from build123d import *

# Parameters (mm, degrees)
SKETCH_W                     = 43.9
SKETCH_H                     = 43.9
SKETCH_W_2                   = 40.7
SKETCH_H_2                   = 40.7
PAD_DEPTH                    = 135
SKETCH001_W                  = 43.9
SKETCH001_H                  = 43.9
PAD001_DEPTH                 = 1.6
PAD002_DEPTH                 = 11.5
PAD002_POLARPATTERN_2_DEPTH  = 11.5
PAD002_POLARPATTERN_3_DEPTH  = 11.5
PAD002_POLARPATTERN_4_DEPTH  = 11.5
SKETCH003_W                  = 43.9
SKETCH003_H                  = 43.9
SKETCH003_W_2                = 35.9
SKETCH003_H_2                = 35.9
PAD003_DEPTH                 = 3.2
PAD004_DEPTH                 = 20
POCKET_DEPTH                 = 21.6
PAD004_LINEARPATTERN_2_DEPTH = 20
POCKET_LINEARPATTERN_2_DEPTH = 21.6


with BuildPart() as part:
    # Sketch → Pad (new body)
    with BuildSketch(Plane.XZ):
        Rectangle(SKETCH_W, SKETCH_H)
        Rectangle(SKETCH_W_2, SKETCH_H_2, mode=Mode.SUBTRACT)
    extrude(amount=PAD_DEPTH)

    # Sketch001 → Pad001 (join)
    with BuildSketch(Plane.XZ):
        Rectangle(SKETCH001_W, SKETCH001_H)
    extrude(amount=-PAD001_DEPTH)

    # Sketch002 → Pad002 (join)
    with BuildSketch(Plane.XZ.offset(135)):
        with BuildLine():
            ThreePointArc((-14.31, 21.95), (-12.21, 19.85), (-10.11, 21.95))
            Line((-14.31, 21.95), (-10.11, 21.95))
        make_face()
    pad002 = extrude(amount=-PAD002_DEPTH)

    # Sketch002 PolarPattern 2 → Pad002 PolarPattern 2 (add)
    with BuildSketch(Plane(origin=(0, -135, 0), x_dir=(0, 0, 1), z_dir=(0, -1, 0))):
        with BuildLine():
            ThreePointArc((-14.31, 21.95), (-12.21, 19.85), (-10.11, 21.95))
            Line((-14.31, 21.95), (-10.11, 21.95))
        make_face()
    pad002_polarpattern_2 = extrude(amount=-PAD002_POLARPATTERN_2_DEPTH)

    # Sketch002 PolarPattern 3 → Pad002 PolarPattern 3 (add)
    with BuildSketch(Plane(origin=(0, -135, 0), x_dir=(-1, 0, 0), z_dir=(0, -1, 0))):
        with BuildLine():
            ThreePointArc((-14.31, 21.95), (-12.21, 19.85), (-10.11, 21.95))
            Line((-14.31, 21.95), (-10.11, 21.95))
        make_face()
    pad002_polarpattern_3 = extrude(amount=-PAD002_POLARPATTERN_3_DEPTH)

    # Sketch002 PolarPattern 4 → Pad002 PolarPattern 4 (add)
    with BuildSketch(Plane(origin=(0, -135, 0), x_dir=(0, 0, -1), z_dir=(0, -1, 0))):
        with BuildLine():
            ThreePointArc((-14.31, 21.95), (-12.21, 19.85), (-10.11, 21.95))
            Line((-14.31, 21.95), (-10.11, 21.95))
        make_face()
    pad002_polarpattern_4 = extrude(amount=-PAD002_POLARPATTERN_4_DEPTH)

    # Mirrored: Pad002, Pad002 PolarPattern 2, Pad002 PolarPattern 3, Pad002 PolarPattern 4 across Sketch002 V_Axis
    add(pad002.mirror(Plane(origin=(0, -135, 0), x_dir=(0, -1, 0), z_dir=(1, 0, 0))))
    add(pad002_polarpattern_2.mirror(Plane(origin=(0, -135, 0), x_dir=(0, -1, 0), z_dir=(1, 0, 0))))
    add(pad002_polarpattern_3.mirror(Plane(origin=(0, -135, 0), x_dir=(0, -1, 0), z_dir=(1, 0, 0))))
    add(pad002_polarpattern_4.mirror(Plane(origin=(0, -135, 0), x_dir=(0, -1, 0), z_dir=(1, 0, 0))))

    # Sketch003 → Pad003 (join)
    with BuildSketch(Plane.XZ.offset(123.5)):
        Rectangle(SKETCH003_W, SKETCH003_H)
        Rectangle(SKETCH003_W_2, SKETCH003_H_2, mode=Mode.SUBTRACT)
    extrude(amount=-PAD003_DEPTH)

    # Sketch004 → Pad004 (join)
    with BuildSketch(Plane.YZ.offset(21.95)):
        with BuildLine():
            ThreePointArc((-110.154, 15.896), (-97.154, 2.896), (-84.154, 15.896))
            Line((-110.154, 15.896), (-84.154, 15.896))
        make_face()
    pad004 = extrude(amount=PAD004_DEPTH)

    # Sketch005 → Pocket (cut)
    with BuildSketch(Plane.YZ.offset(41.95)):
        with BuildLine():
            ThreePointArc((-108.441161, 14.296), (-97.154, 4.496), (-85.866839, 14.296))
            Line((-108.441161, 14.296), (-85.866839, 14.296))
        make_face()
    pocket = extrude(amount=-POCKET_DEPTH, mode=Mode.SUBTRACT)

    # Sketch004 LinearPattern 2 → Pad004 LinearPattern 2 (add)
    with BuildSketch(Plane(origin=(21.95, 80.69, 0), x_dir=(0, 1, 0), z_dir=(1, 0, 0))):
        with BuildLine():
            ThreePointArc((-110.154, 15.896), (-97.154, 2.896), (-84.154, 15.896))
            Line((-110.154, 15.896), (-84.154, 15.896))
        make_face()
    pad004_linearpattern_2 = extrude(amount=PAD004_LINEARPATTERN_2_DEPTH)

    # Sketch005 LinearPattern 2 → Pocket LinearPattern 2 (cut)
    with BuildSketch(Plane(origin=(41.95, 80.69, 0), x_dir=(0, 1, 0), z_dir=(1, 0, 0))):
        with BuildLine():
            ThreePointArc((-108.441161, 14.296), (-97.154, 4.496), (-85.866839, 14.296))
            Line((-108.441161, 14.296), (-85.866839, 14.296))
        make_face()
    pocket_linearpattern_2 = extrude(amount=-POCKET_LINEARPATTERN_2_DEPTH, mode=Mode.SUBTRACT)

    # Mirrored001: Pad004, Pocket, Pad004 LinearPattern 2, Pocket LinearPattern 2 across YZ
    add(pad004.mirror(Plane.YZ))
    add(pocket.mirror(Plane.YZ), mode=Mode.SUBTRACT)
    add(pad004_linearpattern_2.mirror(Plane.YZ))
    add(pocket_linearpattern_2.mirror(Plane.YZ), mode=Mode.SUBTRACT)


solid = part.part
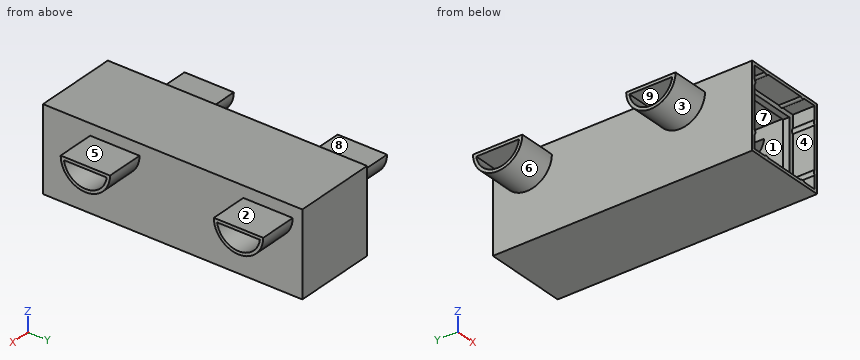
Could you check a few things on this model? Use its own coordinates, in mm. Face numbers are marked on the shaded views. A direction names the side the tool comes from. Coordinates: 2 decimals unless noted, no trailing zeros. Order: outer loops, then holes, each group sorted by start corner. A loop starts at its lowest first (then second) coordinate and runs counter-clockwise, first axis right, second up.
Q1. Suppose I cut it at B-B on z = 0. Please give me the cut outline in (x, y), and give its area (3 significant figures).
Q2. Which directions (+Z, -Z, +X, -X, +Y, -Y) give clear straight access to the entire face, cutting with the end or side of a thin tool? Please do the marked faces 5, 6, 7, 8 and 9.
Q3. Thinking about a two-plate mould opening in Z: for the marked faces 1, 2, 3 and 4, which applies, released by +Z, released by -Z, zero draft, split by the parting line, or undercut?
Q4. Suppose I cut it at D-D on x = -5. Please give me the cut outline in (y, z).
Q5. Please list where these lines run through material, in increasing order: L1, parallel to X at y = -47, z = -0.5; L2, parallel to Y at x = -28, z = 9.5.
Q6. Suppose I cut it at A-A on x = -25. Please give me the cut outline in (y, z), and give its area (3 significant figures).
Q7. Will these pins go through, and if not, where does the flat tip stop? pin 1 (2 mm diameter, centred on y = -131.5, z = 18.5, fed in from -X); pin 2 (1.5 mm diameter, centred on x = 15.5, z = -10, fed in from -Y); pin 3 (9 mm diameter, centred on y = -130.5, z = -1.5, fed in from +X).
Q8. Suppose I cut it at C-C on y = -21.5. Please give me the cut outline in (x, z), and give its area (3 significant figures).
Answer:
1. outline: (-21.95, -135) - (-20.35, -135) - (-20.35, -123.5) - (-17.95, -123.5) - (-17.95, -120.3) - (-20.35, -120.3) - (-20.35, 0) - (20.35, 0) - (20.35, -120.3) - (17.95, -120.3) - (17.95, -123.5) - (20.35, -123.5) - (20.35, -135) - (21.95, -135) - (21.95, 1.6) - (-21.95, 1.6) - close
1. area: 518 mm2
2. face 5: +Z, +X, +Y, -Y
2. face 6: -Z, -X
2. face 7: none
2. face 8: +Z, -X, +Y, -Y
2. face 9: +X, -X
3. face 1: undercut
3. face 2: released by +Z
3. face 3: released by -Z
3. face 4: undercut
4. outline: (-135, -21.95) - (1.6, -21.95) - (1.6, 21.95) - (-135, 21.95) - (-135, 20.35) - (-123.5, 20.35) - (-123.5, 17.95) - (-120.3, 17.95) - (-120.3, 20.35) - (0, 20.35) - (0, -20.35) - (-120.3, -20.35) - (-120.3, -17.95) - (-123.5, -17.95) - (-123.5, -20.35) - (-135, -20.35) - close
5. L1: x = -21.95 to -20.35, 20.35 to 21.95
5. L2: y = -108.47 to -106.59, -87.72 to -85.84, -27.78 to -25.9, -7.03 to -5.15
6. outline: (-110.15, 15.9) arc R13 ccw to (-84.15, 15.9) - close; (-29.46, 15.9) arc R13 ccw to (-3.46, 15.9) - close; hole (-108.44, 14.3) arc R11.4 ccw to (-85.87, 14.3) - close; hole (-27.75, 14.3) arc R11.4 ccw to (-5.18, 14.3) - close
6. area: 195 mm2
7. pin 1: stops at x = -21.95
7. pin 2: stops at y = 0
7. pin 3: stops at x = 21.95
8. outline: (-41.95, 3.91) - (-21.95, 3.91) - (-21.95, -21.95) - (21.95, -21.95) - (21.95, 3.91) - (41.95, 3.91) - (41.95, 5.67) - (20.35, 5.67) - (20.35, -20.35) - (-20.35, -20.35) - (-20.35, 5.67) - (-41.95, 5.67) - close; (-41.95, 14.3) - (-20.35, 14.3) - (-20.35, 20.35) - (20.35, 20.35) - (20.35, 14.3) - (41.95, 14.3) - (41.95, 15.9) - (21.95, 15.9) - (21.95, 21.95) - (-21.95, 21.95) - (-21.95, 15.9) - (-41.95, 15.9) - close
8. area: 377 mm2
